Source: CAD feature listing. Evaluate the final solid. Frame: model axes, mm. Face numbers are marked on the shaded views. A direction names the side the tool comes from. Coordinates: 2 decimals unless noted, no trailing zeros. Order: outer loops, then holes, each group sorted by start corner. A loop starts at its lowest first (then second) coordinate and runs counter-clockwise, first axis right, second up. Notation, with made-up numbers: (79.25, 17) -> (89.25, 17) arc R10 ccw to (89.25, 27) -> close; hole circle Ø7 at (68, 59). An arc over 180 degrees is marked (long way). Put each result on its own line as item: value.
from build123d import *

# Parameters (mm, degrees)
BOSS_EXTRUDE1_DEPTH = 12
CUT_EXTRUDE1_DEPTH  = 26.98557292
SKETCH4_W           = 40
SKETCH4_H           = 12
BOSS_EXTRUDE2_DEPTH = 10
M4_TAPPED_HOLE1_D   = 3.3


with BuildPart() as part:
    # Sketch3 → Boss-Extrude1 (new body)
    with BuildSketch(Plane.XY):
        with BuildLine():
            Line((9.5, 11.5), (9.5, -11.5))
            ThreePointArc((9.5, -11.5), (0, -21), (-9.5, -11.5))
            Line((-9.5, -11.5), (-9.5, 11.5))
            ThreePointArc((-9.5, 11.5), (0, 21), (9.5, 11.5))
        make_face()
    extrude(amount=BOSS_EXTRUDE1_DEPTH)

    # Sketch1 → Cut-Extrude1 (cut, through all)
    with BuildSketch(Plane.XY):
        with BuildLine():
            Line((4.5, 11.5), (4.5, -11.5))
            ThreePointArc((4.5, -11.5), (0, -16), (-4.5, -11.5))
            Line((-4.5, -11.5), (-4.5, 11.5))
            ThreePointArc((-4.5, 11.5), (0, 16), (4.5, 11.5))
        make_face()
    extrude(amount=CUT_EXTRUDE1_DEPTH, mode=Mode.SUBTRACT)

    # Sketch4 → Boss-Extrude2 (add)
    with BuildSketch(Plane.XY):
        with Locations((29.5, -1)):
            Rectangle(SKETCH4_W, SKETCH4_H)
    extrude(amount=BOSS_EXTRUDE2_DEPTH)

    # M4 Tapped Hole1 (through all)
    with Locations(Plane(origin=(0, -7, 0), x_dir=(-1, 0, 0), z_dir=(0, -1, 0))):
        with Locations((-37, -6)):
            Hole(M4_TAPPED_HOLE1_D / 2)


solid = part.part
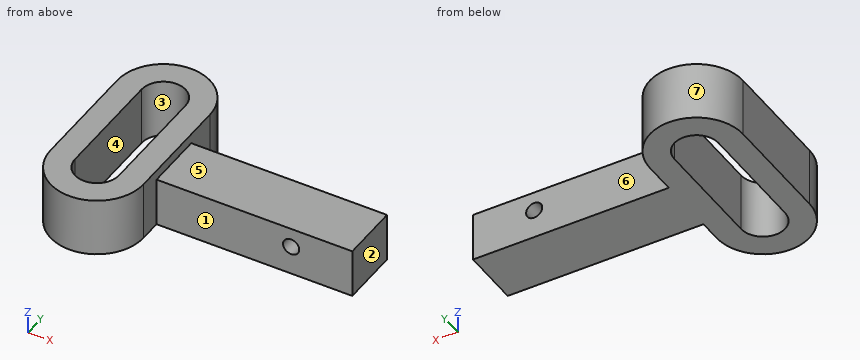
1. First-contact query: pin 1 (2 mm diameter, centred on x = 23.5, z = 7.5, fed in from -Y); pin 2 (3 mm diameter, centred on x = 5.5, z = 5.5, fed in from +Y); pin 3 (3 mm diameter, centred on x = 5.5, z = 9.5, fed in from -Y). Flat tips, straight axial feed; report the tip coordinate or a pass-through.
Numbers:
pin 1: stops at y = -7
pin 2: stops at y = 20.12
pin 3: stops at y = -20.12
2. Cut plane A-A on y = -3.5. Output: boundary loops of the cut face in (x, z), plus the area to 3 significant figures.
Numbers:
outline: (-9.5, 0) -> (-4.5, 0) -> (-4.5, 12) -> (-9.5, 12) -> close; (4.5, 0) -> (49.5, 0) -> (49.5, 10) -> (9.5, 10) -> (9.5, 12) -> (4.5, 12) -> close; hole circle Ø3.3 at (37, 6)
area: 511 mm2
3. Cut plane C-C on x = 0. Output: boundary loops of the cut face in (y, z).
Numbers:
outline: (-21, 0) -> (-16, 0) -> (-16, 12) -> (-21, 12) -> close; (16, 0) -> (21, 0) -> (21, 12) -> (16, 12) -> close
4. Pull-direction query (X, two-part tool) for the marked faces 1, 2 and 3; classes: pulls with the +X half, pulls with the -X half, needs draft (parallel to the pull), parting line crosses it, or undercut.
Numbers:
face 1: needs draft
face 2: pulls with the +X half
face 3: undercut
5. Cut plane D-D on z = 9. Output: boundary loops of the cut face in (x, y).
Numbers:
outline: (-9.5, -11.5) arc R9.5 ccw to (9.5, -11.5) -> (9.5, -7) -> (49.5, -7) -> (49.5, 5) -> (9.5, 5) -> (9.5, 11.5) arc R9.5 ccw to (-9.5, 11.5) -> close; hole (-4.5, -11.5) arc R4.5 ccw to (4.5, -11.5) -> (4.5, 11.5) arc R4.5 ccw to (-4.5, 11.5) -> close
6. Set-up query: the marked faces 4, 5, 6 and 7. Return all of +Z, -Z, +X, -X, +Y, -Y with unobstructed straight access to the full face (end or side cutting, diameter ignored); none if empty.
Numbers:
face 4: +Z, -Z
face 5: +Z, +X, +Y, -Y
face 6: +Z, -Z, +X, +Y
face 7: +Z, -Z, +Y
7. Cut plane B-B on z = 6. Output: boundary loops of the cut face in (x, y), plus the area to 3 significant figures.
Numbers:
outline: (-9.5, -11.5) arc R9.5 ccw to (9.5, -11.5) -> (9.5, -7) -> (35.35, -7) -> (35.35, 5) -> (9.5, 5) -> (9.5, 11.5) arc R9.5 ccw to (-9.5, 11.5) -> close; (38.65, -7) -> (49.5, -7) -> (49.5, 5) -> (38.65, 5) -> close; hole (-4.5, -11.5) arc R4.5 ccw to (4.5, -11.5) -> (4.5, 11.5) arc R4.5 ccw to (-4.5, 11.5) -> close
area: 890 mm2
8. Ray query, line 1 along X through (y, z) = (-2, 6); line 2 along Z through (x, y) = (37, 1.75); line 3 along X through (y, z) = (-4.5, 9). Return the intervals inside material, ascending.
Numbers:
line 1: x = -9.5 to -4.5, 4.5 to 35.35, 38.65 to 49.5
line 2: z = 0 to 4.35, 7.65 to 10
line 3: x = -9.5 to -4.5, 4.5 to 49.5
